Can you work these out from the model? Positions are in its coordinate system, mm. A direction names the side the tool comes from. Round coordinates to 2 decimals unless told otherwise and drop trailing zeros. Loops run counter-clockwise (first coordinate to the right, second up) from the corner with the lowest first, then second, coordinate; pieces in that order, holes last. Notation, with made-up numbers: (-4, -32.5) - (52, -32.5) arc R31 cw to (52, -7.5) - close; hole circle Ø2 at (61, -22). An arc over 180 degrees is marked (long way). Answer as CSV lines item,"result".
```python
from build123d import *

# Parameters (mm, degrees)
EXTRUDE_1_DEPTH     = 6
FILLET_1_R          = 4
SKETCH_2_R          = 4.5
EXTRUDE_2_DEPTH     = 15
SKETCH_4_R          = 6
EXTRUDE_3_DEPTH     = 1
SKETCH_5_R          = 3.5
CUT_EXTRUDE_1_DEPTH = 15
SKETCH_6_W          = 1.5
SKETCH_6_H          = 10.26625424
CUT_EXTRUDE_2_DEPTH = 16.875
CUT_EXTRUDE_3_DEPTH = 0.5


with BuildPart() as part:
    # 草圖1 → 填料-伸長1 (new body)
    with BuildSketch(Plane.XY):
        with BuildLine():
            Line((-11.362913376, -0.524237167), (-9.5, -81.325))
            Line((-9.5, -81.325), (9.5, -81.325))
            Line((9.5, -81.325), (11.362913376, -0.524237167))
            Line((11.362913376, -0.524237167), (11.375, 0))
            ThreePointArc((11.375, 0), (0, 11.375), (-11.375, 0))
            Line((-11.375, 0), (-11.362913376, -0.524237167))
        make_face()
    extrude(amount=EXTRUDE_1_DEPTH)

    # 圓角1
    fillet_1_edges = [part.edges().sort_by_distance(p)[0] for p in [
        (9.5, -81.325, 3),
        (-9.5, -81.325, 3),
    ]]
    fillet(fillet_1_edges, radius=FILLET_1_R)

    # 草圖2 → 填料-伸長2 (add)
    with BuildSketch(Plane.XY.offset(6)):
        Circle(SKETCH_2_R)
    extrude(amount=EXTRUDE_2_DEPTH)

    # 草圖4 → 填料-伸長3 (add)
    with BuildSketch(Plane.XY.offset(6)):
        Circle(SKETCH_4_R)
    extrude(amount=EXTRUDE_3_DEPTH)

    # 草圖5 → 除料-伸長1 (cut)
    with BuildSketch(Plane.XY.offset(21)):
        Circle(SKETCH_5_R)
    extrude(amount=-CUT_EXTRUDE_1_DEPTH, mode=Mode.SUBTRACT)

    # 草圖6 → 除料-伸長2 (cut, through all)
    with BuildSketch(Plane(origin=(0, -4.5, 0), x_dir=(-1, 0, 0), z_dir=(0, -1, 0))):
        with Locations((0, -15.86687288)):
            Rectangle(SKETCH_6_W, SKETCH_6_H)
    extrude(amount=-CUT_EXTRUDE_2_DEPTH, mode=Mode.SUBTRACT)

    # 草圖7 → 除料-伸長3 (cut)
    with BuildSketch(Plane(origin=(0, 0, 0), x_dir=(-1, 0, 0), z_dir=(0, 0, -1))):
        with BuildLine():
            Line((-10.913887181, -20), (10.913887181, -20))
            Line((10.913887181, -20), (11.375, 0))
            ThreePointArc((11.375, 0), (0, 11.375), (-11.375, 0))
            Line((-11.375, 0), (-10.913887181, -20))
        make_face()
    extrude(amount=-CUT_EXTRUDE_3_DEPTH, mode=Mode.SUBTRACT)


solid = part.part
```
Q1. If I drill on line 1 along X through (y, z) = (0, 9.75); line 2 along Z through (x, y) = (-0.5, -68), over which ranges is the centre line in solid material (lowest first)? Write a range as [from, to].
Checks:
line 1,"[-4.5, -3.5], [3.5, 4.5]"
line 2,"[0, 6]"
Q2. We'd pull the mould along X, two halves only. Please class faces 1 (the cylindrical face through (1.615, -3.105, 13.605)), 2 (the cylindrical face through (-5.994, 0.264, 6.493)), 3 (the flat face through (0, 0, 6)), 4 (the flat face through (0, -34, 6)): pulls with the +X half, pulls with the -X half, needs draft (parallel to the pull), parting line crosses it, or undercut.
Checks:
face 1,"undercut"
face 2,"parting line crosses it"
face 3,"undercut"
face 4,"needs draft"
Q3. Imagine slicing it at B-B (y = -31). Write out the boundary of the cut face in (x, z).
Checks:
outline,"(-10.66, 0) - (10.66, 0) - (10.66, 6) - (-10.66, 6) - close"
Q4. I'm going to push flat-ended pins straight in: pin 1 Ø8 at (x, z) = (-3.5, 18) entering from +Y; pin 2 Ø6.5 at (x, y) = (0, 0) entering from +Z; pin 3 Ø12 at (y, z) = (-15, 4.5) entering from -X. Where does each tip first touch, or does it pass through?
Checks:
pin 1,"y = 4.44"
pin 2,"z = 6"
pin 3,"x = -11.17"
Q5. Imagine slicing it at C-C (y = -57). Write out the boundary of the cut face in (x, z), then the cut area to 3 significant figures.
Checks:
outline,"(-10.06, 0) - (10.06, 0) - (10.06, 6) - (-10.06, 6) - close"
area,"121 mm²"
Q6. Imagine slicing it at A-A (z = 18). Write out the boundary of the cut face in (x, y).
Checks:
outline,"(-0.75, -4.44) - (-0.75, -3.42) arc R3.5 cw to (-0.75, 3.42) - (-0.75, 4.44) arc R4.5 ccw to start; (0.75, -4.44) arc R4.5 ccw to (0.75, 4.44) - (0.75, 3.42) arc R3.5 cw to (0.75, -3.42) - close"
Q7. On a 3-axis mill with a long thin cutter (end or side, diameter ignored), from which of +Z, -Z, +X, -X, +Y, -Y can I reach the whole of each face in a straight line? I mean faces 5 (the flat face through (0, -4, 0.5)), 6 (the flat face through (-1.4, 4.5, 7)), 7 (the flat face through (0, -50, 0)). Say none if no direction works.
Checks:
face 5,"-Z, +X, -X, +Y"
face 6,"+Z"
face 7,"-Z, +X, -X, +Y, -Y"
